Study the drawing (mm; zero at the part's minimum x, y, z) and answer. A direction names the side the tool comes from. Round coordinates to 2 decimals unless told otherwise and drop trailing zeros. Loops run counter-clockwise (first coordinate to the right, second up) from the corner with the lowest first, then second, coordinate; pieces in that order, holes last. Notation, with made-up numbers: (6.5, 74) - (53.5, 74) arc R21 cw to (53.5, 86) - close; hole circle Ø9 at (-17, 1.25). An arc over 180 degrees is marked (long way). Use CSV: the item, a comma, the result in double quotes. Start each with the question number.
1. A tool of negligible diameter and unlimited length cuts with its end or side. For the marked faces 1, 2 and 3, from which of +Z, -Z, +X, -X, +Y, -Y can it reach the whole face along a straight path? Write none if from no direction.
2. Determine the mould class of the marked faces 4, 5 and 6 for opening direction X: +X half, -X half, draft (parallel to the pull), parting line (faces both ways), or undercut.
3. Given pin 1 Ø0.6 at (x, y) = (21.5, 2) entering from +Z (1 decimal); pin 2 Ø0.6 at (y, z) = (3, 20) entering from +X (1 decimal); pin 3 Ø1.1 at (y, z) = (2.5, 17.5) entering from -X, each flat-ended and moving along its own axis, determine where each tip first touches the part or whether it passes through.
4. Find section A-A (x = 7). Give the vertices of the cut face in (y, z).
5. Consider line 1 along Z through (x, y) = (7, 4.75); line 2 along Z through (x, y) = (9.5, 3) (1 decimal); line 3 along X through (y, z) = (2, 2.5) (1 decimal). Determine where each line is inside the solid, lowest interval first.
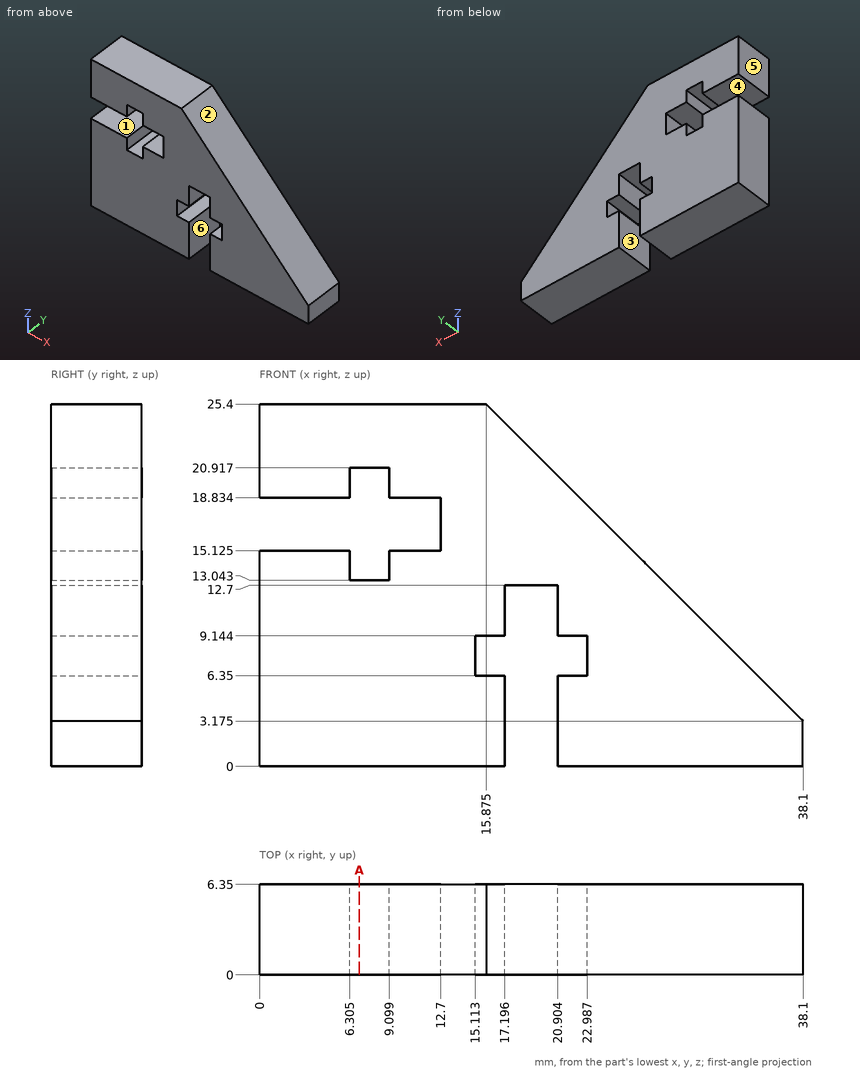
Filled sheet:
1,face 1,"-X, +Y, -Y"
1,face 2,"+Z, +X, +Y, -Y"
1,face 3,"-Z, +Y, -Y"
2,face 4,"draft"
2,face 5,"-X half"
2,face 6,"undercut"
3,pin 1,"stops at z = 20.1"
3,pin 2,"stops at x = 21.6"
3,pin 3,"stops at x = 12.7"
4,outline,"(0, 0) - (6.35, 0) - (6.35, 13.04) - (0, 13.04) - close; (0, 20.92) - (6.35, 20.92) - (6.35, 25.4) - (0, 25.4) - close"
5,line 1,"z = 0 to 13.04, 20.92 to 25.4"
5,line 2,"z = 0 to 15.1, 18.8 to 25.4"
5,line 3,"x = 0 to 17.2, 20.9 to 38.1"
